```python
from build123d import *

# Parameters (mm, degrees)
F0_R     = 1
F1_DEPTH = 2
F2_R     = 3
F2_R_2   = 1.5
F3_DEPTH = 10
F4_W     = 3.5
F4_H     = 12.5
F5_DEPTH = 6
F6_DEPTH = 8
F7_R     = 1
F8_DEPTH = 2


with BuildPart() as f1:
    # F0 (on Top) → F1 (new body)
    with BuildSketch(Plane.XY):
        with BuildLine():
            ThreePointArc((0, 3), (0.87868, 0.87868), (3, 0))
            Line((3, 0), (47, 0))
            ThreePointArc((47, 0), (49.12132, 0.87868), (50, 3))
            ThreePointArc((50, 3), (49.12132, 5.12132), (47, 6))
            Line((47, 6), (14, 6))
            ThreePointArc((14, 6), (11.07073, 16.577113), (10, 27.5))
            Line((10, 27.5), (0, 27.5))
            Line((0, 27.5), (0, 6))
            Line((0, 6), (0, 3))
        make_face()
        with Locations((4, 3)):
            Circle(F0_R, mode=Mode.SUBTRACT)
    extrude(amount=F1_DEPTH)

    # F2 (on face) → F3 (join)
    with BuildSketch(Plane.XY.offset(2)):
        with Locations((47, 3)):
            Circle(F2_R)
        with Locations((47, 3)):
            Circle(F2_R_2, mode=Mode.SUBTRACT)
    extrude(amount=F3_DEPTH)

    # F4 (on face) → F5 (join)
    with BuildSketch(Plane.XY.offset(2)):
        with Locations((1.75, 21.25)):
            Rectangle(F4_W, F4_H)
    extrude(amount=F5_DEPTH)

    # F4 (on face) → F6 (join)
    with BuildSketch(Plane.XY.offset(2)):
        with Locations((1.75, 21.25)):
            Rectangle(F4_W, F4_H)
    extrude(amount=F6_DEPTH)

    # F7 (on face) → F8 (join)
    with BuildSketch(Plane.XY.offset(10)):
        with BuildLine():
            Line((3.5, 15), (3.5, 27.5))
            Line((3.5, 27.5), (-16.5, 27.5))
            Line((-16.5, 27.5), (-16.5, 18))
            ThreePointArc((-16.5, 18), (-15.62132, 15.87868), (-13.5, 15))
            Line((-13.5, 15), (3.5, 15))
        make_face()
        with Locations((-10, 19)):
            Circle(F7_R, mode=Mode.SUBTRACT)
    extrude(amount=F8_DEPTH)

    # F9: F1 across face


with BuildPart() as f1_1:
    add(f1.part)
    add(f1.part.mirror(Plane(origin=(-1.261364, 27.5, 7.136364), x_dir=(-1, 0, 0), z_dir=(0, 1, 0))))


solid = f1_1.part
```
Design review of the part built by this model. Coordinates are the model's own, in mm. A direction names the side the tool comes from. Coordinates: 2 decimals unless noted, no trailing zeros. Loops run counter-clockwise (first coordinate to the right, second up) from the corner with the lowest first, then second, coordinate; pieces in that order, holes last. Notation, with made-up numbers: (-12.75, 63.25) - (40.25, 63.25) arc R17 ccw to (40.25, 74.25) - close; hole circle Ø1 at (33.5, 25). An arc over 180 degrees is marked (long way). Use CSV: the item, a comma, the result in double quotes. Start each with the question number.
1) The part is to be moulded in two halves that separate along Y. For faces 1 (the flat face through (48.3, 53.3, 12)), 2 (the flat face through (47, 3, 2)), 3 (the cylindrical face through (-15.64, 39.1, 10.99)), 4 (the cylindrical face through (-15.64, 15.9, 10.99)), say which applies: +Y half, -Y half, draft (parallel to the pull), parting line (faces both ways), or undercut.
2) Tool access review of faces 5 (the flat face through (-8, 27, 10)), 6 (the cylindrical face through (45.8, 52.9, 6.9)), 7 (the flat face through (-1.3, 15, 10.3)), 8 (the flat face through (-1.3, 40, 10.3)), 9 (the cylindrical face through (11.1, 38.57, 0.99)): name each direction out of +Z, -Z, +X, -X, +Y, -Y from which nothing blocks a thin tool from reaching the whole face with its end or side.
3) Consider section A-A on z = 4.5. Write out the cut boundary in (x, y).
4) Wall thickness on L1, parallel to Y at x = 4, z = 0.6; L2, parallel to Y at x = -10, z = 11.2; L3, parallel to X at y = 36, z = 10.85: over which ranges is each line inside the solid? List them lowest first. Write a range as from..to.
5) Consider section C-C on x = -10. Write out the cut boundary in (y, z), then the cut area to 3 significant figures.
6) Consider section B-B on x = 20.5. Write out the cut boundary in (y, z).
7) For pin 1 Ø18 at (x, y) = (-7.5, 26) entering from -Z; pin 2 Ø3 at (x, z) = (4.5, 5) entering from -Y; pin 3 Ø3 at (y, z) = (30, 8.5) entering from +X; pin 4 Ø4 at (y, z) = (9, 2) entering from -X, all flat-tipped, find the tip position at first contact; note any pin that passes through.
8) Consider section D-D on y = 36. Write out the cut boundary in (x, z), then the cut area to 3 significant figures.
Geometry says:
1,face 1,"draft"
1,face 2,"undercut"
1,face 3,"+Y half"
1,face 4,"-Y half"
2,face 5,"-Z, -X, +Y, -Y"
2,face 6,"+Z"
2,face 7,"+Z, +X, -X, -Y"
2,face 8,"+Z, +X, -X, +Y"
2,face 9,"+Z, -Z, +X"
3,outline,"(0, 15) - (3.5, 15) - (3.5, 40) - (0, 40) - close; circle Ø6 at (47, 3); circle Ø6 at (47, 52); hole circle Ø3 at (47, 3); hole circle Ø3 at (47, 52)"
4,L1,"0..2, 4..51, 53..55"
4,L2,"15..18, 20..35, 37..40"
4,L3,"-16.5..-11, -9..3.5"
5,outline,"(15, 10) - (18, 10) - (18, 12) - (15, 12) - close; (20, 10) - (35, 10) - (35, 12) - (20, 12) - close; (37, 10) - (40, 10) - (40, 12) - (37, 12) - close"
5,area,"42.0 mm^2"
6,outline,"(0, 0) - (6, 0) - (6, 2) - (0, 2) - close; (49, 0) - (55, 0) - (55, 2) - (49, 2) - close"
7,pin 1,"z = 0"
7,pin 2,"y = 15"
7,pin 3,"x = 3.5"
7,pin 4,"x = 0"
8,outline,"(-16.5, 10) - (-11, 10) - (-11, 12) - (-16.5, 12) - close; (-9, 10) - (0, 10) - (0, 0) - (10.67, 0) - (10.67, 2) - (3.5, 2) - (3.5, 12) - (-9, 12) - close"
8,area,"85.3 mm^2"
